Geometry check sheet. Reference: the model listing, model coordinates, mm. A direction names the side the tool comes from. Give positions to 0.01 mm unless a question says otherwise; leave off trailing zeros. Write each loop counter-clockwise with the first axis right and the second up, starting at its lowest first coordinate (ties: lowest second). Pieces come first, ordered by that corner, then holes. Notation, with made-up numbers: (69.5, -39.5) -> (122.5, -39.5) arc R6 ccw to (122.5, -34.5) -> close; hole circle Ø5 at (-9.75, 9). An arc over 180 degrees is marked (long way). Write item = value, one per line. Start each with the question number.
1. Cross-section at C-C, the plane y = 2.5. State how many separate pieces and enclosed holes the cut face has, plus the area to 3 significant figures.
2. Cross-section at D-D, the plane z = -17. Record the cut outline in (x, y).
3. Set-up check for faces 1 (the cylindrical face through (38.626, 2.29, -27.533)), 2 (the flat face through (1, 0, 0)): record each of +Z, -Z, +X, -X, +Y, -Y from which the full face is reachable in a straight line by a thin tool's end or side.
4. Mould release check, pull along X, two halves, no side actions. Record for faces 3 (the flat face through (38.5, 1, 0)), 4 (the cylindrical face through (-33.1, 2.96, -26.57)), 5 (the flat face through (-35.5, 3, 0)), 6 (the flat face through (2, -3, 0)): pulls with the +X half, pulls with the -X half, needs draft (parallel to the pull), parting line crosses it, or undercut.
5. Cross-section at B-B, the plane x = -9. Record the cut outline in (y, z).
6. Cross-section at A-A, the plane x = 37.5. Record the cut outline in (y, z), plus the area to 3 significant figures.
7. Depth check by flat-ended pin: P1, Ø3, axis at y = 4, z = -4, coming from the +X side; P2, Ø10, axis at x = -22, z = 23, coming from the +Y side; P3, Ø3, axis at x = 37.5, z = -28, coming from the -Y side. Enter the tip coordinate at first touch or a pass-through.
8. Thickness scan on line 1 along X through (y, z) = (4.5, -28); line 2 along Z through (x, y) = (37.5, 2.75); line 3 along Z through (x, y) = (-34.5, 0.75). Record the ranges inside material, lowest first.
```python
from build123d import *

# Parameters (mm, degrees)
BOSS_EXTRUDE2_DEPTH                               = 3
BOSS_EXTRUDE3_DEPTH                               = 6
FILLET5_R                                         = 2
CSK_FOR_2_FLAT_HEAD_SOCKET_CAP_SCREW1_D           = 2.4384
CSK_FOR_2_FLAT_HEAD_SOCKET_CAP_SCREW1_CSINK_D     = 5.0038
CSK_FOR_2_FLAT_HEAD_SOCKET_CAP_SCREW1_CSINK_ANGLE = 82
FILLET6_R                                         = 2
FILLET7_R                                         = 1


# Some blends are built 0.0001 mm under size
with BuildPart() as part:
    # Sketch3 → Boss-Extrude2 (new body)
    with BuildSketch(Plane.XZ):
        Polygon((-37.5, 31), (40.5, 31), (40.5, 25.5), (38.5, 25.5), (38.5, -25.5), (40.5, -25.5), (40.5, -31), (-37.5, -31), align=None)
    extrude(amount=BOSS_EXTRUDE2_DEPTH)

    # Sketch4 → Boss-Extrude3 (add)
    with BuildSketch(Plane(origin=(0, 0, 0), x_dir=(1, 0, 0), z_dir=(0, 1, 0))):
        Polygon((-37.5, -31), (40.5, -31), (40.5, -25.5), (38.5, -25.5), (38.5, 25.5), (40.5, 25.5), (40.5, 31), (-37.5, 31), align=None)
        Polygon((-32.5, -29), (35, -29), (35, -26), (36.5, -26), (36.5, 26), (35, 26), (35, 29), (-32.5, 29), (-32.5, 26), (-35.5, 26), (-35.5, -26), (-32.5, -26), align=None, mode=Mode.SUBTRACT)
    extrude(amount=BOSS_EXTRUDE3_DEPTH)

    # Fillet5
    # the kernel refuses this fillet: 2 mm, written as the material it takes off along each edge
    with BuildSketch(Plane(origin=(35, 0, 26), x_dir=(0, 0, 1), z_dir=(0, 1, 0))) as fillet5_piece_1:
        with BuildLine():
            CenterArc((1.936491673, 2), FILLET5_R, 194.477512186, 75.522487814)
            Line((0, 1.5), (-0.038729833, 1.49))
            ThreePointArc((-0.038729833, 1.49), (-0.04, 0.75), (-0.04, 0))
            Line((-0.04, 0), (0, -0.04))
            Line((0, -0.04), (1.936491673, -0.04))
            Line((1.936491673, -0.04), (1.936491673, 0))
        make_face()
    extrude(amount=10.841229183, mode=Mode.SUBTRACT)
    with BuildSketch(Plane(origin=(35, 0, -26), x_dir=(1, 0, 0), z_dir=(0, 1, 0))) as fillet5_piece_2:
        with BuildLine():
            CenterArc((2, 1.936491673), FILLET5_R, 180, 75.522487814)
            Line((0, 1.936491673), (-0.04, 1.936491673))
            Line((-0.04, 1.936491673), (-0.04, 0))
            Line((-0.04, 0), (0, -0.04))
            ThreePointArc((0, -0.04), (0.75, -0.04), (1.49, -0.038729833))
            Line((1.49, -0.038729833), (1.5, 0))
        make_face()
    extrude(amount=10.841229183, mode=Mode.SUBTRACT)
    with BuildSketch(Plane(origin=(-32.5, 0, -26), x_dir=(0, 0, -1), z_dir=(0, 1, 0)), Plane(origin=(-32.5, 0, 26), x_dir=(-1, 0, 0), z_dir=(0, 1, 0))) as fillet5_piece_3:
        with BuildLine():
            CenterArc((FILLET5_R, FILLET5_R), FILLET5_R, 180, 90)
            Line((0, FILLET5_R), (-FILLET5_R * 0.02, FILLET5_R))
            Line((-FILLET5_R * 0.02, FILLET5_R), (-FILLET5_R * 0.02, -FILLET5_R * 0.02))
            Line((-FILLET5_R * 0.02, -FILLET5_R * 0.02), (FILLET5_R, -FILLET5_R * 0.02))
            Line((FILLET5_R, -FILLET5_R * 0.02), (FILLET5_R, 0))
        make_face()
    extrude(amount=11, mode=Mode.SUBTRACT)

    # CSK for #2 Flat Head Socket Cap Screw1 (through all)
    with Locations(Plane(origin=(0, -3, 0), x_dir=(-1, 0, 0), z_dir=(0, -1, 0))):
        with Locations((-37.5, 28), (34.5, 28), (34.5, -28), (-37.5, -28)):
            CounterSinkHole(CSK_FOR_2_FLAT_HEAD_SOCKET_CAP_SCREW1_D / 2, CSK_FOR_2_FLAT_HEAD_SOCKET_CAP_SCREW1_CSINK_D / 2, counter_sink_angle=CSK_FOR_2_FLAT_HEAD_SOCKET_CAP_SCREW1_CSINK_ANGLE)

    # Fillet6
    fillet6_edges = [part.edges().sort_by_distance(p)[0] for p in [
        (40.5, 1.5, -31),
        (-37.5, 1.5, -31),
        (-37.5, 1.5, 31),
        (40.5, 1.5, 31),
    ]]
    fillet(fillet6_edges, radius=FILLET6_R)

    # Fillet7
    fillet7_edges = [part.edges().sort_by_distance(p)[0] for p in [
        (38.5, 1.5, -25.5),
        (38.5, 1.5, 25.5),
    ]]
    fillet(fillet7_edges, radius=FILLET7_R)
    fillet7_2_edges = [part.edges().sort_by_distance(p)[0] for p in [
        (40.5, 1.5, -25.5),
        (40.5, 1.5, 25.5),
    ]]
    fillet(fillet7_2_edges, radius=FILLET7_R - 0.0001)  # a hair under: the kernel refuses the full size


solid = part.part
```
Answers:
q1.separate_pieces = 1
q1.enclosed_holes = 5
q1.area = 560 mm^2
q2.outline = (-37.5, -3) -> (38.5, -3) -> (38.5, 6) -> (36.5, 6) -> (36.5, 0) -> (-35.5, 0) -> (-35.5, 6) -> (-37.5, 6) -> close
q3.face_1 = +Y, -Y
q3.face_2 = +Y
q4.face_3 = pulls with the +X half
q4.face_4 = undercut
q4.face_5 = undercut
q4.face_6 = needs draft
q5.outline = (-3, -31) -> (6, -31) -> (6, -29) -> (0, -29) -> (0, 29) -> (6, 29) -> (6, 31) -> (-3, 31) -> close
q6.outline = (-3, -31) -> (6, -31) -> (6, -29.22) -> (-1.52, -29.22) -> (-3, -30.5) -> close; (-3, -25.5) -> (-1.52, -26.78) -> (6, -26.78) -> (6, 26.78) -> (-1.52, 26.78) -> (-3, 25.5) -> close; (-3, 30.5) -> (-1.52, 29.22) -> (6, 29.22) -> (6, 31) -> (-3, 31) -> close
q6.area = 510 mm^2
q7.P1 = 38.5
q7.P2 = 0
q7.P3 = -1.85
q8.line_1 = -37.5 to -35.72, -33.28 to -32.5, 35 to 36.28, 38.72 to 40.5
q8.line_2 = -31 to -29.22, -26.78 to 26.78, 29.22 to 31
q8.line_3 = -31 to -29.22, -26.78 to -26, 26 to 26.78, 29.22 to 31
